Geometry check sheet. Reference: the model listing, model coordinates, mm. A direction names the side the tool comes from. Round coordinates to 2 decimals unless told otherwise and drop trailing zeros. Write each loop counter-clockwise with the first axis right and the second up, starting at its lowest first coordinate (ties: lowest second). Pieces come first, ordered by that corner, then holes. Notation, with made-up numbers: (33.25, -23.5) - (69.25, -23.5) arc R19 ccw to (69.25, -6.5) - close; hole circle Ø4 at (12.25, -1.75). An arc over 180 degrees is marked (long way). Return JSON: item names as keys, results as strings.
```python
from build123d import *

# Parameters (mm, degrees)
BOSS_EXTRUDE1_DEPTH = 6.6
BOSS_EXTRUDE2_REACH = 24.56
SKETCH3_W           = 6.6
SKETCH3_H           = 7.003924561
SKETCH4_R           = 2
CUT_EXTRUDE1_DEPTH  = 15
SKETCH5_R           = 2
BOSS_EXTRUDE3_DEPTH = 6.69


with BuildPart() as part:
    # Sketch2 → Boss-Extrude1 (new body)
    with BuildSketch(Plane.XY):
        Polygon((0, 0), (0, 94.86), (-6.6, 94.86), (-6.6, 5.71), (-22.56, 5.71), (-22.56, 94.86), (-29.16, 94.86), (-29.16, 0), align=None)
    extrude(amount=BOSS_EXTRUDE1_DEPTH)

    # Sketch3 → Boss-Extrude2 (add, up to next)
    with BuildSketch(Plane(origin=(-22.56, 0, 0), x_dir=(0, 0, -1), z_dir=(1, 0, 0)), mode=Mode.PRIVATE) as boss_extrude2_sk1:
        with Locations((-3.3, 91.35803772)):
            Rectangle(SKETCH3_W, SKETCH3_H)
    boss_extrude2_tool1 = extrude(boss_extrude2_sk1.sketch, amount=BOSS_EXTRUDE2_REACH, mode=Mode.PRIVATE) - part.part
    add(boss_extrude2_tool1.solids().sort_by_distance((-22.56, 91.358038, 3.3))[0])

    # Sketch4 → Cut-Extrude1 (cut)
    with BuildSketch(Plane.XY.offset(6.6)):
        with Locations((-3.354353393, 47.428062363)):
            Circle(SKETCH4_R)
        with Locations((-25.771024386, 47.428062363)):
            Circle(SKETCH4_R)
        with Locations((-25.771024386, 3.86)):
            Circle(SKETCH4_R)
        with Locations((-3.354353393, 3.86)):
            Circle(SKETCH4_R)
        with Locations((-25.771024386, 74.86)):
            Circle(SKETCH4_R)
        with Locations((-3.354353393, 74.86)):
            Circle(SKETCH4_R)
    extrude(amount=-CUT_EXTRUDE1_DEPTH, mode=Mode.SUBTRACT)

    # Sketch5 → Boss-Extrude3 (add)
    with BuildSketch(Plane.XY.offset(6.6)):
        with Locations((-25.771024386, 47.428062363)):
            Circle(SKETCH5_R)
        with Locations((-3.354353393, 47.428062363)):
            Circle(SKETCH5_R)
    extrude(amount=-BOSS_EXTRUDE3_DEPTH)


solid = part.part
```
(1) Access from +Z, -Z, +X, -X, +Y, -Y to the whole of each face (thin tool, end or side, straight path). Record for faces 5 (the face through (-15, 87.856, 3)), 6 (the face through (-25, 47, 6.6)).
Response values:
{"face 5": "+Z, -Z", "face 6": "+Z, +X, -X, +Y, -Y"}
(2) Material ranges on line 1 along X through (y, z) = (81, 2.5); line 2 along Y through (x, z) = (-11, 3.5); line 3 along Y through (x, z) = (-4.5, 1), recorded low to high. Write a range as [from, to].
Response values:
{"line 1": "x = [-29.16, -22.56], [-6.6, 0]", "line 2": "y = [0, 5.71], [87.86, 94.86]", "line 3": "y = [0, 2.22], [5.5, 73.22], [76.5, 94.86]"}
(3) Section check D-D, the plane x = -9. Enter the section's corners in (y, z), plus the area to 3 significant figures.
Response values:
{"outline": "(0, 0) - (5.71, 0) - (5.71, 6.6) - (0, 6.6) - close; (87.86, 0) - (94.86, 0) - (94.86, 6.6) - (87.86, 6.6) - close", "area": "83.9 mm^2"}
(4) Section check A-A, the plane y = 3.86. Enter the section's corners in (x, z).
Response values:
{"outline": "(-29.16, 0) - (-27.77, 0) - (-27.77, 6.6) - (-29.16, 6.6) - close; (-23.77, 0) - (-5.35, 0) - (-5.35, 6.6) - (-23.77, 6.6) - close; (-1.35, 0) - (0, 0) - (0, 6.6) - (-1.35, 6.6) - close"}
(5) Gauge pin test, flat ends, axial feed: pin 1 (14.5 mm diameter, centred on x = -20.5, y = 61, fed in from -Z); pin 2 (2.5 mm diameter, centred on x = -25.77, y = 3.86, fed in from -Z). Record the tip position at first contact, or that the pin passes through.
Response values:
{"pin 1": "stops at z = 0", "pin 2": "passes through"}
(6) Section check C-C, the plane y = 74.86. Enter the section's corners in (x, z), plus the area to 3 significant figures.
Response values:
{"outline": "(-29.16, 0) - (-27.77, 0) - (-27.77, 6.6) - (-29.16, 6.6) - close; (-23.77, 0) - (-22.56, 0) - (-22.56, 6.6) - (-23.77, 6.6) - close; (-6.6, 0) - (-5.35, 0) - (-5.35, 6.6) - (-6.6, 6.6) - close; (-1.35, 0) - (0, 0) - (0, 6.6) - (-1.35, 6.6) - close", "area": "34.3 mm^2"}
(7) Release check for a two-part mould opening along Y. For faces 1 (the face through (-23.863, 4.461, 3.346)), 2 (the face through (-26, 47, -0.09)), 3 (the face through (-3.79, 72.91, 3.35)), 4 (the face through (-15, 0, 3)) record: pulls with the +Y half, pulls with the -Y half, needs draft (parallel to the pull), parting line crosses it, or undercut.
Response values:
{"face 1": "undercut", "face 2": "needs draft", "face 3": "undercut", "face 4": "pulls with the -Y half"}
(8) Section check B-B, the plane z = 1.5. Enter the section's corners in (x, y), plus the area to 3 significant figures.
Response values:
{"outline": "(-29.16, 0) - (0, 0) - (0, 94.86) - (-29.16, 94.86) - close; hole circle Ø4 at (-25.77, 3.86); hole circle Ø4 at (-25.77, 74.86); hole (-22.56, 5.71) - (-6.6, 5.71) - (-6.6, 87.86) - (-22.56, 87.86) - close; hole circle Ø4 at (-3.35, 3.86); hole circle Ø4 at (-3.35, 74.86)", "area": "1,400 mm^2"}
